Model file for the job. Use its own axes, mm. A direction names the side the tool comes from. Round coordinates to 2 decimals unless told otherwise and drop trailing zeros. Answer in a Markdown table with one row per item.
from build123d import *

# Parameters (mm, degrees)
SKETCH1_W                        = 14.3
SKETCH1_H                        = 1
SKETCH2_R                        = 12.5
BOSS_EXTRUDE1_DEPTH              = 3.5
F_7_0_7_DIAMETER_HOLE1_D         = 7
F_7_0_7_DIAMETER_HOLE1_DEPTH     = 3.3
SKETCH17_R                       = 3.5
SKETCH17_R_2                     = 3.25
BOSS_EXTRUDE3_DEPTH              = 0.5
SKETCH18_R                       = 6
CUT_EXTRUDE4_DEPTH               = 1
SKETCH19_R                       = 4
BOSS_EXTRUDE4_DEPTH              = 1
CUT_EXTRUDE1_DEPTH               = 1
CUT_EXTRUDE2_DEPTH               = 1
CUT_EXTRUDE3_DEPTH               = 1
F_2_0_2_DIAMETER_HOLE1_D         = 2
F_2_0_2_DIAMETER_HOLE1_DEPTH     = 2.3
CBORE_FOR_M1_6_SHCS1_D           = 2
CBORE_FOR_M1_6_SHCS1_CBORE_D     = 3.62300003
CBORE_FOR_M1_6_SHCS1_CBORE_DEPTH = 2
M2_CLEARANCE_HOLE1_D             = 2.529
M2_CLEARANCE_HOLE1_DEPTH         = 4
CHAMFER1_SIZE                    = 0.5
CHAMFER2_SIZE                    = 0.3
CHAMFER3_SIZE                    = 0.2
CHAMFER4_SIZE                    = 1
FILLET1_R                        = 1


with BuildPart() as part:
    # Sketch1 → Revolve1 (revolve)
    with BuildSketch(Plane(origin=(0, 0, 0), x_dir=(1, 0, 0), z_dir=(0, 1, 0))):
        with Locations((7.15, -9.7)):
            Rectangle(SKETCH1_W, SKETCH1_H)
    revolve(axis=Axis((0, 0, 9.2), (0, 0, 1)))

    # Sketch2 → Boss-Extrude1 (add)
    with BuildSketch(Plane(origin=(0, 0, 9.2), x_dir=(-1, 0, 0), z_dir=(0, 0, -1))):
        with Locations(Location((0, 0, 0), (0, 0, 180))):
            Circle(SKETCH2_R)
    extrude(amount=BOSS_EXTRUDE1_DEPTH)

    # Ø7.0 (7) Diameter Hole1
    with Locations(Plane(origin=(0, 0, 5.7), x_dir=(1, 0, 0), z_dir=(0, 0, -1))):
        with Locations((0, 0)):
            Hole(F_7_0_7_DIAMETER_HOLE1_D / 2, depth=F_7_0_7_DIAMETER_HOLE1_DEPTH)

    # Sketch17 → Boss-Extrude3 (add)
    with BuildSketch(Plane(origin=(0, 0, 9), x_dir=(-1, 0, 0), z_dir=(0, 0, -1))):
        Circle(SKETCH17_R)
        Circle(SKETCH17_R_2, mode=Mode.SUBTRACT)
    extrude(amount=BOSS_EXTRUDE3_DEPTH)

    # Sketch18 → Cut-Extrude4 (cut)
    with BuildSketch(Plane.XY.offset(10.2)):
        Circle(SKETCH18_R)
    extrude(amount=-CUT_EXTRUDE4_DEPTH, mode=Mode.SUBTRACT)

    # Sketch19 → Boss-Extrude4 (add)
    with BuildSketch(Plane.XY.offset(9.2)):
        Circle(SKETCH19_R)
    extrude(amount=BOSS_EXTRUDE4_DEPTH)

    # Sketch6 → Cut-Extrude1 (cut)
    with BuildSketch(Plane.XY.offset(10.2)):
        with BuildLine():
            Line((2.903285774, 10.835210018), (2.070552392, 7.727406725))
            ThreePointArc((2.070552392, 7.727406725), (4.00000006, 6.928203334), (5.656854334, 5.656854334))
            Line((5.656854334, 5.656854334), (7.931924244, 7.931924244))
            ThreePointArc((7.931924244, 7.931924244), (5.60871742, 9.714583538), (2.903285774, 10.835210018))
        make_face()
    extrude(amount=-CUT_EXTRUDE1_DEPTH, mode=Mode.SUBTRACT)

    # Sketch7 → Cut-Extrude2 (cut)
    with BuildSketch(Plane.XY.offset(10.2)):
        with BuildLine():
            Line((7.931924244, -7.931924244), (5.656854334, -5.656854334))
            ThreePointArc((5.656854334, -5.656854334), (4.00000006, -6.928203334), (2.070552392, -7.727406725))
            Line((2.070552392, -7.727406725), (2.903285774, -10.835210018))
            ThreePointArc((2.903285774, -10.835210018), (5.60871742, -9.714583538), (7.931924244, -7.931924244))
        make_face()
    extrude(amount=-CUT_EXTRUDE2_DEPTH, mode=Mode.SUBTRACT)

    # Sketch8 → Cut-Extrude3 (cut)
    with BuildSketch(Plane.XY.offset(10.2)):
        with BuildLine():
            Line((-10.835210018, -2.903285774), (-7.727406725, -2.070552392))
            ThreePointArc((-7.727406725, -2.070552392), (-8.000000119, 0), (-7.727406725, 2.070552392))
            Line((-7.727406725, 2.070552392), (-10.835210018, 2.903285774))
            ThreePointArc((-10.835210018, 2.903285774), (-11.217434841, 0), (-10.835210018, -2.903285774))
        make_face()
    extrude(amount=-CUT_EXTRUDE3_DEPTH, mode=Mode.SUBTRACT)

    # Ø2.0 (2) Diameter Hole1
    with Locations(Plane(origin=(0, 0, 5.7), x_dir=(-1, 0, 0), z_dir=(0, 0, -1))):
        with Locations((-4.5, 7.794228634), (9, 0), (-4.5, -7.794228634)):
            Hole(F_2_0_2_DIAMETER_HOLE1_D / 2, depth=F_2_0_2_DIAMETER_HOLE1_DEPTH)

    # CBORE for M1.6 SHCS1 (through all)
    with Locations(Plane.XY.offset(10.2)):
        with Locations((-4.5, 7.794228634), (-4.5, -7.794228634), (9, 0)):
            CounterBoreHole(CBORE_FOR_M1_6_SHCS1_D / 2, CBORE_FOR_M1_6_SHCS1_CBORE_D / 2, CBORE_FOR_M1_6_SHCS1_CBORE_DEPTH)

    # M2 Clearance Hole1
    with Locations(Plane.XY.offset(10.2)):
        with Locations((7.794228634, -4.5), (-7.794228634, -4.5), (7.794228634, 4.5), (0, -9), (-7.794228634, 4.5), (0, 9)):
            Hole(M2_CLEARANCE_HOLE1_D / 2, depth=M2_CLEARANCE_HOLE1_DEPTH)

    # Chamfer1
    chamfer1_edges = [part.edges().sort_by_distance(p)[0] for p in [
        (-6.311500015, 7.794228634, 10.2),
        (7.188499985, 0, 10.2),
        (-6.311500015, -7.794228634, 10.2),
        (-12.5, 0, 5.7),
    ]]
    chamfer(chamfer1_edges, length=CHAMFER1_SIZE)

    # Chamfer2
    chamfer2_edges = [part.edges().sort_by_distance(p)[0] for p in [
        (-6, 0, 10.2),
        (-14.3, 0, 10.2),
    ]]
    chamfer(chamfer2_edges, length=CHAMFER2_SIZE)

    # Chamfer3
    chamfer3_edges = [part.edges().sort_by_distance(p)[0] for p in [
        (-14.3, 0, 9.2),
    ]]
    chamfer(chamfer3_edges, length=CHAMFER3_SIZE)

    # Chamfer4
    chamfer4_edges = [part.edges().sort_by_distance(p)[0] for p in [
        (-4, 0, 9.2),
    ]]
    chamfer(chamfer4_edges, length=CHAMFER4_SIZE - 0.0001)  # a hair under: the kernel refuses the full size

    # Fillet1
    fillet1_edges = [part.edges().sort_by_distance(p)[0] for p in [
        (2.903285774, 10.835210018, 9.7),
        (7.931924244, 7.931924244, 9.7),
        (5.656854334, 5.656854334, 9.7),
        (2.070552392, 7.727406725, 9.7),
        (7.931924244, -7.931924244, 9.7),
        (2.903285774, -10.835210018, 9.7),
        (2.070552392, -7.727406725, 9.7),
        (5.656854334, -5.656854334, 9.7),
        (-10.835210018, -2.903285774, 9.7),
        (-10.835210018, 2.903285774, 9.7),
        (-7.727406725, 2.070552392, 9.7),
        (-7.727406725, -2.070552392, 9.7),
    ]]
    fillet(fillet1_edges, radius=FILLET1_R)


solid = part.part
1. Saw through at A-A (z = 6.85). State how many separate pieces and enclosed holes the cut face has, and give its area (3 significant figures).
Verdict:
| item | result |
|---|---|
| separate pieces | 1 |
| enclosed holes | 13 |
| area | 403 mm² |
2. Wall check: probe 1 along Y at (x, z) = (0, 8.4); probe 2 along Y at (x, z) = (-8.25, 6.25); probe 3 along X at (y, z) = (8.25, 6.85). Give the ranges that are in metal, low to high.
Verdict:
| item | result |
|---|---|
| probe 1 | y = -12.5 to -10.26, -7.74 to -3.5, 3.5 to 7.74, 10.26 to 12.5 |
| probe 2 | y = -9.39 to -5.68, -3.32 to -0.66, 0.66 to 3.32, 5.68 to 9.39 |
| probe 3 | x = -9.39 to -5.39, -3.61 to -1.02, 1.02 to 3.61, 5.39 to 9.39 |
3. Mould opens along X. For faces 3 (the flat face through (-6, -3, 10.2)), 4 (the cylindrical face through (4.015, -6.92, 9.707)) say: +X half, -X half, draft (parallel to the pull), parting line (faces both ways), or undercut.
Verdict:
| item | result |
|---|---|
| face 3 | draft |
| face 4 | undercut |
4. Pin check, flat tips, straight feed: pin 1 (3 mm diameter, centred on x = -5, y = 7.5, fed in from +Z); pin 2 (2.5 mm diameter, centred on x = -4.5, y = 7.79, fed in from +Z); pin 3 (1.6 mm diameter, centred on x = -9, y = 0, fed in from +Z). Stop position of each tip, or through.
Verdict:
| item | result |
|---|---|
| pin 1 | stops at z = 9.97 |
| pin 2 | stops at z = 8.2 |
| pin 3 | stops at z = 9.2 |
5. Tool access for faces 1 (the cylindrical face through (-3.233, 1.341, 7.12)), 2 (the flat face through (5, 8, 9.2)): list every direction of +Z, -Z, +X, -X, +Y, -Y with a clear straight run to the whole face (end or side of a thin tool).
Verdict:
| item | result |
|---|---|
| face 1 | -Z |
| face 2 | +Z |
